The model under review builds one solid part; all positions refer to its coordinate system, in mm. Round coordinates to 2 decimals unless told otherwise and drop trailing zeros. Write each loop counter-clockwise with the first axis right and the second up, starting at its lowest first coordinate (ties: lowest second). Pieces come first, ordered by that corner, then holes.
Item 1: Add section A-A (z = 4.5). Give the boundary of the cut face in (x, y).
Item 2: To check wall thickness, follow L1, parallel to Y at x = -15, z = 4.5; L2, parallel to Y at x = 18.5, z = 1.25; L3, parallel to X at y = 62, z = 5.5. State the ranges of each line that lie inside material, in increasing order.
Item 3: Add section D-D (y = -2). Give the boundary of the cut face in (x, z), plus the area to 3 significant figures.
Item 4: Add section C-C (x = 15). Give the boundary of the cut face in (y, z).
Item 5: Add section B-B (y = 25). Give the boundary of the cut face in (x, z).
Item 6: Clearance check with flat-ended pins moving along their axes: pin 1 Ø1 at (y, z) = (12, 5.5) entering from +X; pin 2 Ø1 at (y, z) = (59.5, 5.5) entering from -X (3 decimals); pin 3 Ø4.5 at (x, y) = (-15, 25) entering from +Z; pin 4 Ø1 at (y, z) = (39.5, 2.5) entering from +X. State where each tip first meets the part, or that it passes through.
```python
from build123d import *

# Parameters (mm, degrees)
F1_R     = 2.6
F1_R_2   = 1.75
F2_DEPTH = 8


with BuildPart() as f2:
    # F1 (on Top) → F2 (new body)
    with BuildSketch(Plane.XY):
        with BuildLine():
            ThreePointArc((-71.3722397476, 66.4353312303), (-39.3316918026, 59.4869377058), (-25, 30))
            ThreePointArc((-25, 30), (-33.0130622942, 6.8316918026), (-53.6277602524, -6.4353312303))
            ThreePointArc((-53.6277602524, -6.4353312303), (0, 0), (53.6277602524, -6.4353312303))
            ThreePointArc((53.6277602524, -6.4353312303), (26.0646687697, 38.8722397476), (71.3722397476, 66.4353312303))
            ThreePointArc((71.3722397476, 66.4353312303), (0, 75), (-71.3722397476, 66.4353312303))
        make_face()
        with Locations((-15, 25)):
            Circle(F1_R, mode=Mode.SUBTRACT)
        with Locations((0, 25)):
            Circle(F1_R, mode=Mode.SUBTRACT)
        with Locations((15, 25)):
            Circle(F1_R, mode=Mode.SUBTRACT)
        with BuildLine():
            ThreePointArc((-53.6277602524, -6.4353312303), (-33.0130622942, 6.8316918026), (-25, 30))
            ThreePointArc((-25, 30), (-39.3316918026, 59.4869377058), (-71.3722397476, 66.4353312303))
            ThreePointArc((-71.3722397476, 66.4353312303), (-98.9353312303, 21.1277602524), (-53.6277602524, -6.4353312303))
        make_face()
        with Locations((-50, 20)):
            Circle(F1_R_2, mode=Mode.SUBTRACT)
        with BuildLine():
            ThreePointArc((100, 30), (91.9869377058, 53.1683081974), (71.3722397476, 66.4353312303))
            ThreePointArc((71.3722397476, 66.4353312303), (26.0646687697, 38.8722397476), (53.6277602524, -6.4353312303))
            ThreePointArc((53.6277602524, -6.4353312303), (85.6683081974, 0.5130622942), (100, 30))
        make_face()
        with Locations((50, 20)):
            Circle(F1_R_2, mode=Mode.SUBTRACT)
        with Locations((0, 25)):
            Circle(F1_R)
        with Locations((-50, 20)):
            Circle(F1_R_2)
        with Locations((50, 20)):
            Circle(F1_R_2)
    extrude(amount=F2_DEPTH)


solid = f2.part
```
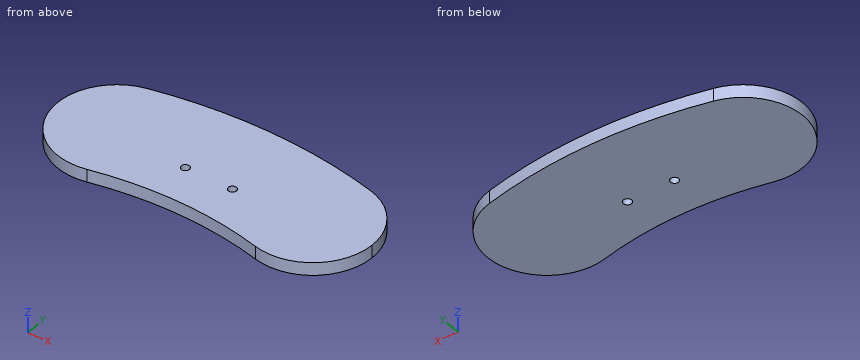
Numbers:
1. outline: (-71.37, 66.44) arc R37.5 ccw to (-53.63, -6.44) arc R226.67 cw to (53.63, -6.44) arc R37.5 ccw to (71.37, 66.44) arc R301.67 ccw to start; hole circle Ø5.2 at (-15, 25); hole circle Ø5.2 at (15, 25)
2. L1: y = -0.5 to 22.4, 27.6 to 74.63
2. L2: y = -0.76 to 74.43
2. L3: x = -82.05 to 82.05
3. outline: (-82.05, 0) - (-30.04, 0) - (-30.04, 8) - (-82.05, 8) - close; (30.04, 0) - (82.05, 0) - (82.05, 8) - (30.04, 8) - close
3. area: 832 mm2
4. outline: (-0.5, 0) - (22.4, 0) - (22.4, 8) - (-0.5, 8) - close; (27.6, 0) - (74.63, 0) - (74.63, 8) - (27.6, 8) - close
5. outline: (-99.67, 0) - (-17.6, 0) - (-17.6, 8) - (-99.67, 8) - close; (-12.4, 0) - (12.4, 0) - (12.4, 8) - (-12.4, 8) - close; (17.6, 0) - (99.67, 0) - (99.67, 8) - (17.6, 8) - close
6. pin 1: stops at x = 95.67
6. pin 2: stops at x = -86.275
6. pin 3: passes through
6. pin 4: stops at x = 98.9
